Verification items for the finished model (mm, model axes). Face numbers are marked on the shaded views. A direction names the side the tool comes from. Coordinates: 2 decimals unless noted, no trailing zeros. Order: outer loops, then holes, each group sorted by start corner. A loop starts at its lowest first (then second) coordinate and runs counter-clockwise, first axis right, second up. Notation, with made-up numbers: M 11.25,47.25 L 53.25,47.25 A32 cw 53.25,79.25 Z; hole C 12,16 d2. An arc over 180 degrees is marked long. Write item = value, one per line.
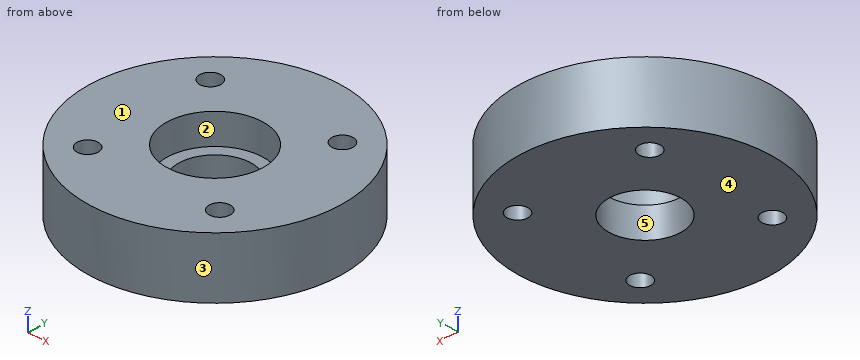
```python
from build123d import *

# Parameters (mm, degrees)
SKETCH1_R           = 21
BOSS_EXTRUDE1_DEPTH = 10
SKETCH2_R           = 6
CUT_EXTRUDE1_DEPTH  = 32.336879232
SKETCH3_R           = 8
CUT_EXTRUDE2_DEPTH  = 5
SKETCH4_R           = 1.75
CUT_EXTRUDE3_DEPTH  = 32.336879232


with BuildPart() as part:
    # Sketch1 → Boss-Extrude1 (new body)
    with BuildSketch(Plane.XY):
        Circle(SKETCH1_R)
    extrude(amount=BOSS_EXTRUDE1_DEPTH)

    # Sketch2 → Cut-Extrude1 (cut, through all)
    with BuildSketch(Plane.XY.offset(10)):
        Circle(SKETCH2_R)
    extrude(amount=-CUT_EXTRUDE1_DEPTH, mode=Mode.SUBTRACT)

    # Sketch3 → Cut-Extrude2 (cut)
    with BuildSketch(Plane.XY.offset(10)):
        Circle(SKETCH3_R)
    extrude(amount=-CUT_EXTRUDE2_DEPTH, mode=Mode.SUBTRACT)

    # Sketch4 → Cut-Extrude3 (cut, through all)
    with BuildSketch(Plane.XY.offset(10)):
        with Locations((-11, 11)):
            Circle(SKETCH4_R)
        with Locations(Location((11, 11, 0), (0, 0, 180))):
            Circle(SKETCH4_R)
        with Locations((11, -11)):
            Circle(SKETCH4_R)
        with Locations(Location((-11, -11, 0), (0, 0, 180))):
            Circle(SKETCH4_R)
    extrude(amount=-CUT_EXTRUDE3_DEPTH, mode=Mode.SUBTRACT)


solid = part.part
```
Item 1: Sectioned sample at B-B, the plane y = 5.5. Enter the section's corners in (x, z), then the cut area to 3 significant figures.
Report:
outline = M -20.27,0 L -2.4,0 L -2.4,5 L -5.81,5 L -5.81,10 L -20.27,10 Z; M 2.4,0 L 20.27,0 L 20.27,10 L 5.81,10 L 5.81,5 L 2.4,5 Z
area = 323 mm^2
Item 2: Sectioned sample at A-A, the plane x = 0. Enter the section's corners in (y, z).
Report:
outline = M -21,0 L -6,0 L -6,5 L -8,5 L -8,10 L -21,10 Z; M 6,0 L 21,0 L 21,10 L 8,10 L 8,5 L 6,5 Z
Item 3: Sectioned sample at D-D, the plane x = 11. Enter the section's corners in (y, z), then the cut area to 3 significant figures.
Report:
outline = M -17.89,0 L -12.75,0 L -12.75,10 L -17.89,10 Z; M -9.25,0 L 9.25,0 L 9.25,10 L -9.25,10 Z; M 12.75,0 L 17.89,0 L 17.89,10 L 12.75,10 Z
area = 288 mm^2
Item 4: Release check for a two-part mould opening along X. For the marked faces 3, 4 and 5 record: pulls with the +X half, pulls with the -X half, needs draft (parallel to the pull), parting line crosses it, or undercut.
Report:
face_3 = parting line crosses it
face_4 = needs draft
face_5 = undercut
Item 5: Sectioned sample at C-C, the plane z = 1.25. Enter the section's corners in (x, y).
Report:
outline = C 0,0 d42; hole C -11,-11 d3.5; hole C -11,11 d3.5; hole C 0,0 d12; hole C 11,-11 d3.5; hole C 11,11 d3.5
Item 6: Gauge pin test, flat ends, axial feed: pin 1 (3 mm diameter, centred on y = 13, z = 6, fed in from -X); pin 2 (4 mm diameter, centred on y = -16.5, z = 5.5, fed in from -X); pin 3 (3 mm diameter, centred on y = 5.5, z = 8.5, fed in from +X). Record the tip position at first contact, or that the pin passes through.
Report:
pin_1 = -17.57
pin_2 = -15.19
pin_3 = 20.62
Item 7: Scan lines: L1, parallel to Y at x = 0, z = 6.75; L2, parallel to X at y = -9.5, z = 4; L3, parallel to Y at x = 10, z = 8.5. Record each from-to range of solid material in increasing order. Write a range as from..to.
Report:
L1 = -21..-8, 8..21
L2 = -18.73..-11.9, -10.1..10.1, 11.9..18.73
L3 = -18.47..-12.44, -9.56..9.56, 12.44..18.47
Item 8: Tool access check on the marked faces 1 and 2. Record the directions out of +Z, -Z, +X, -X, +Y, -Y that give a thin tool (end or side, any length) a straight path to the whole face; none if there is none.
Report:
face_1 = +Z, +X, -X, +Y, -Y
face_2 = +Z
